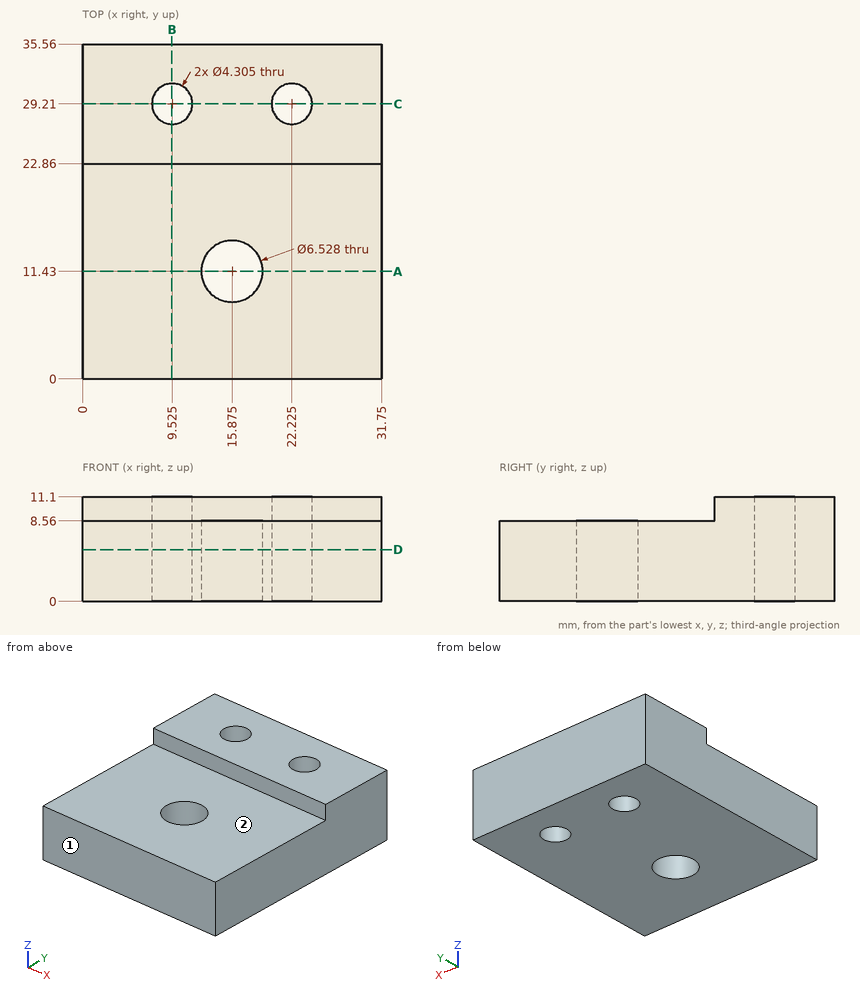
Verification items for this drawing (mm, ordinates from the low corner). A direction names the side the tool comes from. Round coordinates to 2 decimals unless told otherwise and drop trailing zeros. Order: outer loops, then holes, each group sorted by start corner. A loop starts at its lowest first (then second) coordinate and runs counter-clockwise, first axis right, second up. Notation, with made-up numbers: (-3.5, 17) - (34.5, 17) arc R22 ccw to (34.5, 45) - close; hole circle Ø7 at (32, 17.5). An arc over 180 degrees is marked (long way). Use CSV: the item, a comma, the result in double quotes. Start each with the question number.
1) Section check A-A, the plane y = 11.43. Record the cut outline in (x, z).
2) Access from +Z, -Z, +X, -X, +Y, -Y to the whole of each face (thin tool, end or side, straight path). Record for the marked faces 1 and 2.
3) Section check B-B, the plane x = 9.5. Record the cut outline in (y, z), plus the area to 3 significant figures.
4) Go/stop test with flat-tipped pins: P1, Ø5, axis at x = 15.875, y = 11.43, coming from the +Z side; P2, Ø1.3, axis at x = 17, z = 9.5, coming from the -Y side. Record where each tip stops, or that it passes through.
5) Section check C-C, the plane y = 29.21. Record the cut outline in (x, z), plus the area to 3 significant figures.
6) Thickness scan on L1, parallel to Y at x = 9.5, z = 5; L2, parallel to X at y = 30.5, z = 1.25; L3, parallel to Z at x = 30.5, y = 12.5. Record the ranges inside material, lowest first.
7) Section check D-D, the plane z = 5.5. State how many separate pieces and enclosed holes the cut face has, plus the area to 3 significant figures.
Answers:
1,outline,"(0, 0) - (12.61, 0) - (12.61, 8.56) - (0, 8.56) - close; (19.14, 0) - (31.75, 0) - (31.75, 8.56) - (19.14, 8.56) - close"
2,face 1,"+Z, -Z, +X, -X, -Y"
2,face 2,"+Z, +X, -X, -Y"
3,outline,"(0, 0) - (27.06, 0) - (27.06, 11.1) - (22.86, 11.1) - (22.86, 8.56) - (0, 8.56) - close; (31.36, 0) - (35.56, 0) - (35.56, 11.1) - (31.36, 11.1) - close"
3,area,"289 mm²"
4,P1,"passes through"
4,P2,"stops at y = 22.86"
5,outline,"(0, 0) - (7.37, 0) - (7.37, 11.1) - (0, 11.1) - close; (11.68, 0) - (20.07, 0) - (20.07, 11.1) - (11.68, 11.1) - close; (24.38, 0) - (31.75, 0) - (31.75, 11.1) - (24.38, 11.1) - close"
5,area,"257 mm²"
6,L1,"y = 0 to 27.06, 31.36 to 35.56"
6,L2,"x = 0 to 7.8, 11.25 to 20.5, 23.95 to 31.75"
6,L3,"z = 0 to 8.56"
7,separate pieces,"1"
7,enclosed holes,"3"
7,area,"1,070 mm²"
